```python
from build123d import *

# Parameters (mm, degrees)
SKETCH1_W            = 161.925
SKETCH1_H            = 118.745
SKETCH1_R            = 1.55
SKETCH1_R_2          = 1.5
BOSS_EXTRUDE1_DEPTH  = 1.56
SKETCH2_W            = 20
SKETCH2_H            = 10.4775
SKETCH2_W_2          = 15.3
SKETCH2_H_2          = 7.62
SKETCH2_W_3          = 11
SKETCH2_H_3          = 6.0325
SKETCH2_W_4          = 15.5
SKETCH2_H_4          = 6.6675
BOSS_EXTRUDE2_DEPTH  = 5
SKETCH4_W            = 17.8
SKETCH4_H            = 15.24
BOSS_EXTRUDE3_DEPTH  = 9.4
SKETCH5_W            = 15.24
SKETCH5_H            = 14.4
SKETCH5_R            = 6.5
CUT_EXTRUDE1_DEPTH   = 4
SKETCH7_W            = 15.5
SKETCH7_H            = 13.335
CUT_EXTRUDE3_DEPTH   = 2.75
SKETCH8_W            = 12.835
SKETCH8_H            = 1.75
CUT_EXTRUDE4_DEPTH   = 15
SKETCH9_W            = 14
SKETCH9_H            = 12.065
BOSS_EXTRUDE4_DEPTH  = 6.4
SKETCH10_W           = 10.065
SKETCH10_H           = 7.4
CUT_EXTRUDE5_DEPTH   = 13
SKETCH11_W           = 9.07
SKETCH11_H           = 2
BOSS_EXTRUDE5_DEPTH  = 13
BOSS_EXTRUDE6_DEPTH  = 5
BOSS_EXTRUDE8_DEPTH  = 4
SKETCH38_W           = 31.093633867
SKETCH38_H           = 25.604360888
CUT_EXTRUDE14_DEPTH  = 10
SKETCH39_W           = 16.3
SKETCH39_H           = 18.54
BOSS_EXTRUDE9_DEPTH  = 12.7
SKETCH40_W           = 1.16
SKETCH40_H           = 1.16
SKETCH40_H_2         = 12.7
BOSS_EXTRUDE10_DEPTH = 2.03
SKETCH41_W           = 13.67
SKETCH41_H           = 9.91
BOSS_EXTRUDE11_DEPTH = 3.51
CUT_EXTRUDE15_DEPTH  = 111.727077745
SKETCH43_W           = 9
SKETCH43_H           = 40.34
BOSS_EXTRUDE12_DEPTH = 10.16
CUT_EXTRUDE16_DEPTH  = 8.66
SKETCH46_W           = 120
SKETCH46_H           = 9.5
SKETCH46_W_2         = 7
SKETCH46_H_2         = 10
SKETCH46_W_3         = 7.773635701
SKETCH46_W_4         = 12
SKETCH46_H_3         = 18
SKETCH46_H_4         = 2.178592617
BOSS_EXTRUDE14_DEPTH = 3
BOSS_EXTRUDE15_DEPTH = 13
SKETCH49_W           = 4
SKETCH49_H           = 7.4
BOSS_EXTRUDE16_DEPTH = 7.31
SKETCH50_R           = 1.75
BOSS_EXTRUDE17_DEPTH = 1.5


with BuildPart() as part:
    # Sketch1 → Boss-Extrude1 (new body)
    with BuildSketch(Plane(origin=(0, 0, 0), x_dir=(1, 0, 0), z_dir=(0, 1, 0))):
        with Locations((10.228253106, -2.102894012)):
            Rectangle(SKETCH1_W, SKETCH1_H)
        with Locations(Location((-42.794246894, -44.860394012, 0), (0, 0, 90))):
            Circle(SKETCH1_R, mode=Mode.SUBTRACT)
        with Locations(Location((-61.844246894, 51.554605988, 0), (0, 0, 90))):
            Circle(SKETCH1_R, mode=Mode.SUBTRACT)
        with Locations(Location((70.205753106, 13.139605988, 0), (0, 0, 90))):
            Circle(SKETCH1_R_2, mode=Mode.SUBTRACT)
        with Locations(Location((-16.294246894, -3.500394012, 0), (0, 0, 90))):
            Circle(SKETCH1_R_2, mode=Mode.SUBTRACT)
        with Locations(Location((76.205753106, -43.860394012, 0), (0, 0, 90))):
            Circle(SKETCH1_R_2, mode=Mode.SUBTRACT)
    extrude(amount=BOSS_EXTRUDE1_DEPTH)

    # Sketch2 → Boss-Extrude2 (add)
    with BuildSketch(Plane(origin=(0, 1.56, 0), x_dir=(1, 0, 0), z_dir=(0, 1, 0))):
        with Locations((-60.734246894, -42.901644012)):
            Rectangle(SKETCH2_W, SKETCH2_H)
        with Locations((-60.734246894, -53.379144012)):
            Rectangle(SKETCH2_W, SKETCH2_H)
        with Locations((-63.084246894, -30.360394012)):
            Rectangle(SKETCH2_W_2, SKETCH2_H_2)
        with Locations((-63.084246894, -22.740394012)):
            Rectangle(SKETCH2_W_2, SKETCH2_H_2)
        Polygon((-70.734246894, -34.170394012), (-70.734246894, -26.550394012), (-70.734246894, -18.930394012), (-73.234246894, -18.930394012), (-73.234246894, -34.170394012), align=None)
        with Locations((-65.234246894, 6.945855988)):
            Rectangle(SKETCH2_W_3, SKETCH2_H_3)
        Polygon((-70.734246894, -2.102894012), (-70.734246894, 3.929605988), (-70.734246894, 9.962105988), (-73.734246894, 9.962105988), (-73.734246894, -2.102894012), align=None)
        with Locations((-65.234246894, 0.913355988)):
            Rectangle(SKETCH2_W_3, SKETCH2_H_3)
        with Locations((-62.984246894, 37.743355988)):
            Rectangle(SKETCH2_W_4, SKETCH2_H_4)
        with Locations((-62.984246894, 31.075855988)):
            Rectangle(SKETCH2_W_4, SKETCH2_H_4)
    extrude(amount=BOSS_EXTRUDE2_DEPTH)

    # Sketch4 → Boss-Extrude3 (add)
    with BuildSketch(Plane(origin=(0, 6.56, 0), x_dir=(1, 0, 0), z_dir=(0, 1, 0))):
        with Locations((-64.334246894, -26.550394012)):
            Rectangle(SKETCH4_W, SKETCH4_H)
    extrude(amount=BOSS_EXTRUDE3_DEPTH)

    # Sketch5 → Cut-Extrude1 (cut)
    with BuildSketch(Plane.ZY.offset(73.234246894)):
        with Locations((26.550394012, 8.76)):
            Rectangle(SKETCH5_W, SKETCH5_H)
        with Locations((26.550394012, 8.76)):
            Circle(SKETCH5_R, mode=Mode.SUBTRACT)
    extrude(amount=-CUT_EXTRUDE1_DEPTH, mode=Mode.SUBTRACT)

    # Sketch7 → Cut-Extrude3 (cut)
    with BuildSketch(Plane(origin=(0, 6.56, 0), x_dir=(1, 0, 0), z_dir=(0, 1, 0))):
        with Locations((-62.984246894, 34.409605988)):
            Rectangle(SKETCH7_W, SKETCH7_H)
    extrude(amount=-CUT_EXTRUDE3_DEPTH, mode=Mode.SUBTRACT)

    # Sketch8 → Cut-Extrude4 (cut)
    with BuildSketch(Plane.ZY.offset(70.734246894)):
        with Locations((-34.409605988, 2.685)):
            Rectangle(SKETCH8_W, SKETCH8_H)
    extrude(amount=-CUT_EXTRUDE4_DEPTH, mode=Mode.SUBTRACT)

    # Sketch9 → Boss-Extrude4 (add)
    with BuildSketch(Plane(origin=(0, 6.56, 0), x_dir=(1, 0, 0), z_dir=(0, 1, 0))):
        with Locations((-66.734246894, 3.929605988)):
            Rectangle(SKETCH9_W, SKETCH9_H)
    extrude(amount=BOSS_EXTRUDE4_DEPTH)

    # Sketch10 → Cut-Extrude5 (cut)
    with BuildSketch(Plane.ZY.offset(73.734246894)):
        with Locations((-3.929605988, 7.26)):
            Rectangle(SKETCH10_W, SKETCH10_H)
    extrude(amount=-CUT_EXTRUDE5_DEPTH, mode=Mode.SUBTRACT)

    # Sketch11 → Boss-Extrude5 (add)
    with BuildSketch(Plane.ZY.offset(60.734246894)):
        with Locations((-3.927105988, 6.46)):
            Rectangle(SKETCH11_W, SKETCH11_H)
    extrude(amount=BOSS_EXTRUDE5_DEPTH)

    # Sketch12 → Boss-Extrude6 (add)
    with BuildSketch(Plane(origin=(0, 6.56, 0), x_dir=(1, 0, 0), z_dir=(0, 1, 0))):
        Polygon((-70.734246894, -58.617894012), (-71.734246894, -58.617894012), (-71.734246894, -60.117894012), (-73.734246894, -60.117894012), (-73.806970959, -36.162894012), (-71.734246894, -36.162894012), (-71.734246894, -37.662894012), (-70.734246894, -37.662894012), align=None)
    extrude(amount=-BOSS_EXTRUDE6_DEPTH)

    # Sketch13 → Boss-Extrude8 (add)
    with BuildSketch(Plane(origin=(0, 6.56, 0), x_dir=(1, 0, 0), z_dir=(0, 1, 0))):
        Polygon((-50.734246894, -37.662894012), (-50.734246894, -58.617894012), (-71.734246894, -58.617894012), (-71.734246894, -60.117894012), (-73.734246894, -60.117894012), (-73.806970959, -36.162894012), (-71.734246894, -36.162894012), (-71.734246894, -37.662894012), align=None)
    extrude(amount=BOSS_EXTRUDE8_DEPTH)

    # Sketch38 → Cut-Extrude14 (cut)
    with BuildSketch(Plane(origin=(0, 1.56, 0), x_dir=(1, 0, 0), z_dir=(0, 1, 0))):
        with Locations((-64.389815501, -47.792725567)):
            Rectangle(SKETCH38_W, SKETCH38_H)
    extrude(amount=CUT_EXTRUDE14_DEPTH, mode=Mode.SUBTRACT)

    # Sketch39 → Boss-Extrude9 (add)
    with BuildSketch(Plane(origin=(0, 1.56, 0), x_dir=(1, 0, 0), z_dir=(0, 1, 0))):
        with Locations((-62.584246894, -48.145394012)):
            Rectangle(SKETCH39_W, SKETCH39_H)
    extrude(amount=BOSS_EXTRUDE9_DEPTH)

    # Sketch40 → Boss-Extrude10 (add)
    with BuildSketch(Plane.ZY.offset(70.734246894)):
        with Locations((38.295394012, 14.84)):
            Rectangle(SKETCH40_W, SKETCH40_H)
        Polygon((38.875394012, 15.42), (38.875394012, 14.26), (57.415394012, 14.26), (57.415394012, 1.56), (58.575394012, 1.56), (58.575394012, 15.42), align=None)
        with Locations((38.295394012, 7.91)):
            Rectangle(SKETCH40_W, SKETCH40_H_2)
        Polygon((57.415394012, 14.26), (38.875394012, 14.26), (38.875394012, 1.56), (37.715394012, 1.56), (37.715394012, 0.4), (57.415394012, 0.4), (57.415394012, 1.56), align=None)
        with Locations((57.995394012, 0.98)):
            Rectangle(SKETCH40_W, SKETCH40_H)
    extrude(amount=BOSS_EXTRUDE10_DEPTH)

    # Sketch41 → Boss-Extrude11 (add)
    with BuildSketch(Plane.ZY.offset(72.764246894)):
        with Locations((48.145394012, 7.91)):
            Rectangle(SKETCH41_W, SKETCH41_H)
    extrude(amount=BOSS_EXTRUDE11_DEPTH)

    # Sketch42 → Cut-Extrude15 (cut, through all)
    with BuildSketch(Plane(origin=(0, 12.865, 0), x_dir=(1, 0, 0), z_dir=(0, 1, 0))):
        Polygon((-72.764246894, -41.310394012), (-76.274246894, -54.980394012), (-76.274246894, -41.310394012), align=None)
    extrude(amount=-CUT_EXTRUDE15_DEPTH, mode=Mode.SUBTRACT)

    # Sketch43 → Boss-Extrude12 (add)
    with BuildSketch(Plane(origin=(0, 1.56, 0), x_dir=(1, 0, 0), z_dir=(0, 1, 0))):
        with Locations((61.345753106, -3.060394012)):
            Rectangle(SKETCH43_W, SKETCH43_H)
    extrude(amount=BOSS_EXTRUDE12_DEPTH)

    # Sketch44 → Cut-Extrude16 (cut)
    with BuildSketch(Plane(origin=(0, 11.72, 0), x_dir=(1, 0, 0), z_dir=(0, 1, 0))):
        Polygon((57.845753106, -0.810394012), (56.845753106, -0.810394012), (56.845753106, -5.310394012), (57.845753106, -5.310394012), (57.845753106, -22.230394012), (64.845753106, -22.230394012), (64.845753106, 16.109605988), (57.845753106, 16.109605988), align=None)
    extrude(amount=-CUT_EXTRUDE16_DEPTH, mode=Mode.SUBTRACT)

    # Sketch46 → Boss-Extrude14 (add)
    with BuildSketch(Plane.XZ):
        with Locations((19.265753106, -47.519605988)):
            Rectangle(SKETCH46_W, SKETCH46_H)
        with Locations((-67.234246894, -19.269605988)):
            Rectangle(SKETCH46_W_2, SKETCH46_H_2)
        with Locations((-41.847429044, -19.269605988)):
            Rectangle(SKETCH46_W_3, SKETCH46_H_2)
        with Locations((-64.734246894, -2.132030476)):
            Rectangle(SKETCH46_W_4, SKETCH46_H_3)
        with Locations((-45.018245774, 0.319690321)):
            Rectangle(SKETCH46_W_2, SKETCH46_H_4)
    extrude(amount=BOSS_EXTRUDE14_DEPTH)

    # Sketch47 → Boss-Extrude15 (add)
    with BuildSketch(Plane.ZY.offset(73.734246894)):
        Polygon((-6.929605988, 10.96), (-8.962105988, 8.9275), (-8.962105988, 10.96), align=None)
        Polygon((-0.929605988, 10.96), (1.102894012, 8.9275), (1.102894012, 10.96), align=None)
    extrude(amount=-BOSS_EXTRUDE15_DEPTH)

    # Sketch49 → Boss-Extrude16 (add)
    with BuildSketch(Plane(origin=(0, 1.56, 0), x_dir=(1, 0, 0), z_dir=(0, 1, 0))):
        with Locations((-68.734246894, 18.124605988)):
            Rectangle(SKETCH49_W, SKETCH49_H)
    extrude(amount=BOSS_EXTRUDE16_DEPTH)

    # Sketch50 → Boss-Extrude17 (add)
    with BuildSketch(Plane.ZY.offset(70.734246894)):
        with Locations(Location((-18.124605988, 5.87, 0), (0, 0, 180))):
            Circle(SKETCH50_R)
    extrude(amount=BOSS_EXTRUDE17_DEPTH)


solid = part.part
```
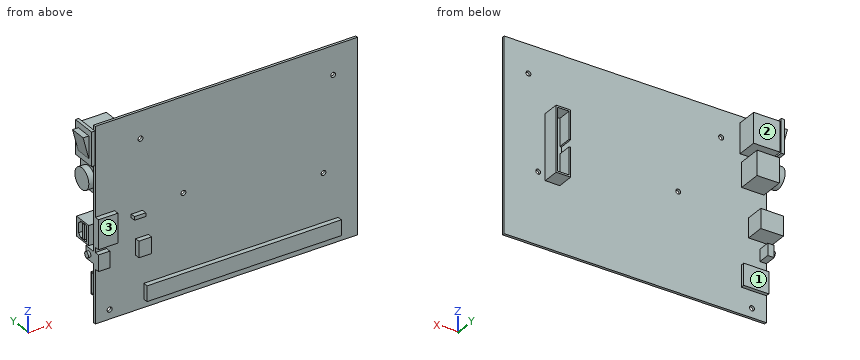
Geometry: final body of the model. Coordinates: model frame, mm. Face numbers are marked on the shaded views. A direction names the side the tool comes from. Give positions to 0.01 mm unless a question says otherwise; leave off trailing zeros. Loops run counter-clockwise (first coordinate to the right, second up) from the corner with the lowest first, then second, coordinate; pieces in that order, holes last. Notation, with made-up numbers: (0.25, -14.5) - (36.25, -14.5) arc R14 ccw to (36.25, -10.5) - close; hole circle Ø2 at (55, -19). An arc over 180 degrees is marked (long way). Answer as CSV lines item,"result". Start each with the question number.
(1) Section query C-C (x = 81.5). Output: boundary loops of the cut face in (y, z).
(2) Section query A-A (x = -25). Output: boundary loops of the cut face in (y, z), and give its area (3 significant figures).
(3) Section query B-B (z = 31). Output: boundary loops of the cut face in (x, y), and give its area (3 significant figures).
(4) Reachability of the marked faces 1, 2 and 3 from +Z, -Z, +X, -X, +Y, -Y: full face, straight path, thin tool, end or side. Return the list, or none.
(5) Pin query (flat end, axial travel): P1, Ø10, axis at y = 8, z = 45, coming from the +X side; P2, Ø1.8, axis at y = 5.5, z = -18.5, coming from the -X side; P3, Ø4, axis at y = 6.5, z = 10, coming from the +X side; P4, Ø3, axis at x = -49.5, y = 3, coming from the -Z side. Return the tip coordinate at first contact, or that it passes through.
(6) Ray query, line 1 along X through (y, z) = (8.75, -6); line 2 along Z through (x, y) = (-59, 7); line 3 along X through (y, z) = (2.5, -13). Return the intervals inside material, ascending. Write a range as [from, to].
Worked answers:
1,outline,"(0, -57.27) - (1.56, -57.27) - (1.56, 61.48) - (0, 61.48) - close"
2,outline,"(-3, -52.27) - (0, -52.27) - (0, -57.27) - (1.56, -57.27) - (1.56, 61.48) - (0, 61.48) - (0, -42.77) - (-3, -42.77) - close"
2,area,"214 mm^2"
3,outline,"(-73.23, 4.02) - (-69.23, 4.02) - (-69.23, 1.56) - (-70.73, 1.56) - (-70.73, 0) - (91.19, 0) - (91.19, 1.56) - (-55.43, 1.56) - (-55.43, 15.96) - (-69.23, 15.96) - (-69.23, 13.5) - (-73.23, 13.5) - close"
3,area,"489 mm^2"
4,face 1,"-Z, +X, -X, +Y"
4,face 2,"+Z, +X, +Y"
4,face 3,"+Z, -Z, +X, -X, -Y"
5,P1,"stops at x = -54.43"
5,P2,"stops at x = -72.23"
5,P3,"stops at x = 65.85"
5,P4,"stops at z = -57.27"
6,line 1,"x = [-60.73, -59.73], [56.85, 57.85], [64.85, 65.85]"
6,line 2,"z = [18.93, 34.17], [38.88, 57.42]"
6,line 3,"x = [56.85, 65.85]"
